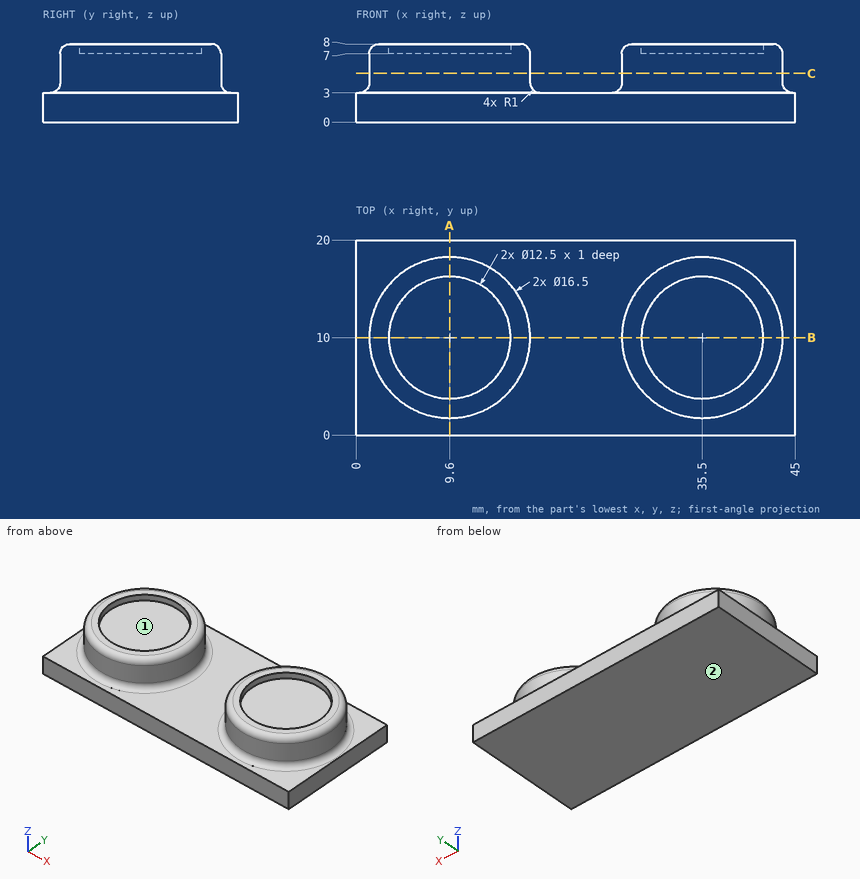
Source: three-view drawing plus pictorial views. Frame: mm from the lowest corner of the part. Coordinates: 2 decimals unless noted, no trailing zeros. Write each loop counter-clockwise with the first axis right and the second up, starting at its lowest first coordinate (ties: lowest second). Pieces come first, ordered by that corner, then holes. Notation, with made-up numbers: (89.5, -12.5) -> (148.5, -12.5) arc R20 cw to (148.5, 24.5) -> close; hole circle Ø4 at (23.5, 80.5). An arc over 180 degrees is marked (long way). Write each question's results on one line, items separated by ' | '.
Item 1: Section query A-A on x = 9.6. Return loops of the section in (y, z).
Conclusion:
outline: (0, 0) -> (20, 0) -> (20, 3) -> (19.25, 3) arc R1 cw to (18.25, 4) -> (18.25, 7) arc R1 ccw to (17.25, 8) -> (16.25, 8) -> (16.25, 7) -> (3.75, 7) -> (3.75, 8) -> (2.75, 8) arc R1 ccw to (1.75, 7) -> (1.75, 4) arc R1 cw to (0.75, 3) -> (0, 3) -> close
Item 2: Section query C-C on z = 5. Return loops of the section in (x, y).
Conclusion:
outline: circle Ø16.5 at (9.6, 10); circle Ø16.5 at (35.5, 10)
Item 3: Section query B-B on y = 10. Return loops of the section in (x, z), plus the area to 3 significant figures.
Conclusion:
outline: (0, 0) -> (45, 0) -> (45, 3) -> (44.75, 3) arc R1 cw to (43.75, 4) -> (43.75, 7) arc R1 ccw to (42.75, 8) -> (41.75, 8) -> (41.75, 7) -> (29.25, 7) -> (29.25, 8) -> (28.25, 8) arc R1 ccw to (27.25, 7) -> (27.25, 4) arc R1 cw to (26.25, 3) -> (18.85, 3) arc R1 cw to (17.85, 4) -> (17.85, 7) arc R1 ccw to (16.85, 8) -> (15.85, 8) -> (15.85, 7) -> (3.35, 7) -> (3.35, 8) -> (2.35, 8) arc R1 ccw to (1.35, 7) -> (1.35, 4) arc R1 cw to (0.35, 3) -> (0, 3) -> close | area: 275 mm^2
Item 4: Material intervals for probe 1 along Y at (x, z) = (9.6, 7.35); probe 2 along X at (y, z) = (9, 4); probe 3 along Z at (x, y) = (20, 8.5), sorted ascending.
Conclusion:
probe 1: y = 1.81 to 3.75, 16.25 to 18.19 | probe 2: x = 1.41 to 17.79, 27.31 to 43.69 | probe 3: z = 0 to 3
Item 5: Mould query, pull axis X, two halves, no side actions, for the marked faces 1 and 2. Classes: +X half, -X half, draft (parallel to the pull), parting line (faces both ways), or undercut.
Conclusion:
face 1: undercut | face 2: draft
